```python
from build123d import *

# Parameters (mm, degrees)
F0_R     = 2.3
F0_W     = 48.5
F0_H     = 28.5
F0_W_2   = 6
F0_H_2   = 23.5
F0_W_3   = 39.2
F0_H_3   = 6
F0_H_4   = 12.9
F1_DEPTH = 6


with BuildPart() as f1:
    # F0 (on Top) → F1 (new body)
    with BuildSketch(Plane.XY):
        Polygon((-62.5, 35), (-82.3, 35), (-82.3, 11.5), (-82.3, -2.5), (-79.3, -2.5), (-79.3, 0.5), (-76.3, 0.5), (-76.3, -2.5), (-72.8, -2.5), (-72.8, -4.5), (-72.8, -6.5), (-76.3, -6.5), (-76.3, -9.5), (-79.3, -9.5), (-79.3, -6.5), (-82.3, -6.5), (-82.3, -35), (82.3, -35), (82.3, -21), (82.3, -8.1), (82.3, 0.5), (79.3, 0.5), (79.3, -2.5), (76.3, -2.5), (76.3, 0.5), (72.8, 0.5), (72.8, 4.5), (76.3, 4.5), (76.3, 7.5), (79.3, 7.5), (79.3, 4.5), (82.3, 4.5), (82.3, 12.85), (82.3, 25.75), (82.3, 35), (61.3, 35), (22.1, 35), (1.45, 35), (1.45, 32), (4.45, 32), (4.45, 29), (1.45, 29), (1.45, 25.5), (-2.55, 25.5), (-2.55, 29), (-5.55, 29), (-5.55, 32), (-2.55, 32), (-2.55, 35), (-23.3, 35), align=None)
        with Locations((38.636842, -17.724174)):
            Circle(F0_R, mode=Mode.SUBTRACT)
        with Locations((38.636842, 2.150826)):
            Rectangle(F0_W, F0_H, mode=Mode.SUBTRACT)
        with Locations((38.636842, 22.025826)):
            Circle(F0_R, mode=Mode.SUBTRACT)
        with Locations((-85.3, 23.25)):
            Rectangle(F0_W_2, F0_H_2)
        with Locations((-42.9, 38)):
            Rectangle(F0_W_3, F0_H_3)
        with Locations((41.7, 38)):
            Rectangle(F0_W_3, F0_H_3)
        with Locations((85.3, 19.3)):
            Rectangle(F0_W_2, F0_H_4)
        with Locations((85.3, -14.55)):
            Rectangle(F0_W_2, F0_H_4)
    extrude(amount=F1_DEPTH)


solid = f1.part
```
Work out the finished part from the listing and answer in its coordinate system (mm). A direction names the side the tool comes from. Round coordinates to 2 decimals unless told otherwise and drop trailing zeros. Loops run counter-clockwise (first coordinate to the right, second up) from the corner with the lowest first, then second, coordinate; pieces in that order, holes last. Notation, with made-up numbers: M 1.25,48.5 L 34.25,48.5 A21 ccw 34.25,75.5 Z; hole C 12.25,57.25 d2. An arc over 180 degrees is marked long. One line per question, with ' | ' between items.
Q1. Find section C-C, the plane z = 4.8. State how many separate pieces and enclosed holes the cut face has, then the cut area to 3 significant figures.
Conclusion:
separate pieces: 1 | enclosed holes: 3 | area: 10,700 mm2
Q2. Find section D-D, the plane x = -19.5. Give the vertices of the cut face in (y, z), then the cut area to 3 significant figures.
Conclusion:
outline: M -35,0 L 35,0 L 35,6 L -35,6 Z | area: 420 mm2
Q3. A tool of negligible diameter and unlimited length cuts with its end or side. For faces 1 (the flat face through (-4, 32, 3)), 2 (the flat face through (85, -21, 3)), 3 (the flat face through (-75, -6.5, 3)), 4 (the flat face through (85, -8.1, 3)), 5 (the flat face through (-82.3, 5, 3)), from which of +Z, -Z, +X, -X, +Y, -Y can it reach the whole face along a straight path? Write none if from no direction.
Conclusion:
face 1: +Z, -Z | face 2: +Z, -Z, +X, -Y | face 3: +Z, -Z, -X | face 4: +Z, -Z, +X | face 5: +Z, -Z, -X, -Y
Q4. Each of these flat-tipped pins is pushed along its axis until it touches: pin 1 Ø6 at (x, y) = (26, -11.5) entering from +Z; pin 2 Ø2 at (y, z) = (-27, 1.5) entering from -X; pin 3 Ø1.5 at (y, z) = (6.5, 3.5) entering from +X; pin 4 Ø3 at (x, z) = (0.5, 2.5) entering from +Y. Where does it stop, or does it pass through?
Conclusion:
pin 1: stops at z = 6 | pin 2: stops at x = -82.3 | pin 3: stops at x = 82.3 | pin 4: stops at y = 35
Q5. Find section B-B, the plane y = -29. Give the vertices of the cut face in (x, z), then the cut area to 3 significant figures.
Conclusion:
outline: M -82.3,0 L 82.3,0 L 82.3,6 L -82.3,6 Z | area: 988 mm2
Q6. Find section A-A, the plane x = 17.5. Give the vertices of the cut face in (y, z), then the cut area to 3 significant figures.
Conclusion:
outline: M -35,0 L -12.1,0 L -12.1,6 L -35,6 Z; M 16.4,0 L 35,0 L 35,6 L 16.4,6 Z | area: 249 mm2
Q7. Consider line 1 along X through (y, z) = (6, 1.95); line 2 along X through (y, z) = (-4.5, 2.1); line 3 along X through (y, z) = (-8, 4). Determine where each line is inside the solid, lowest interval first. Write a range as from..to.
Conclusion:
line 1: x = -82.3..14.39, 62.89..76.3, 79.3..82.3 | line 2: x = -72.8..14.39, 62.89..82.3 | line 3: x = -82.3..-79.3, -76.3..14.39, 62.89..82.3
Q8. The mould has two halves that part along X. Classify faces 6 (the flat face through (41, 41, 3)), 7 (the flat face through (-79.3, -8, 3)), 8 (the flat face through (1.45, 27, 3)), 9 (the flat face through (82.3, 9, 3)): +X half, -X half, draft (parallel to the pull), parting line (faces both ways), or undercut.
Conclusion:
face 6: draft | face 7: undercut | face 8: undercut | face 9: +X half
